Input: part model. Units: mm. Frame: model coordinates. Face numbers are marked on the shaded views. A direction names the side the tool comes from. Give positions to 0.01 mm unless a question says otherwise; leave off trailing zeros. Order: outer loops, then holes, each group sorted by start corner. A loop starts at its lowest first (then second) coordinate and runs counter-clockwise, first axis right, second up. Notation, with made-up numbers: M -17,-36.5 L -1,-36.5 A14 cw -1,-18.5 Z; hole C 40,53 d2. An arc over 180 degrees is marked long. Use a Markdown table: item, result.
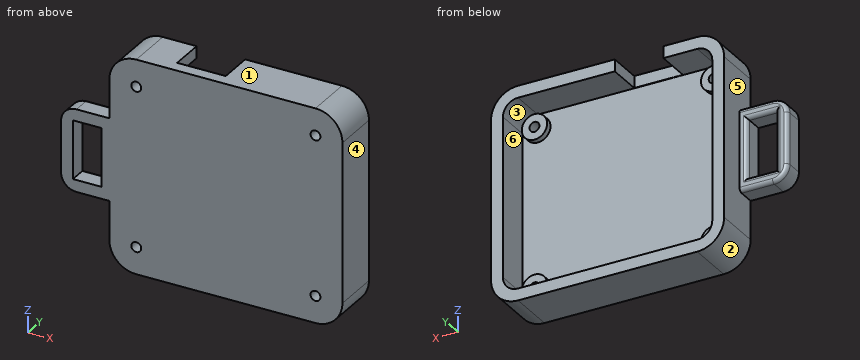
from build123d import *

# Parameters (mm, degrees)
BOSS_EXTRUDE1_DEPTH = 3
CUT_EXTRUDE1_REACH  = 77.661
SKETCH1_3_R         = 1.25
BOSS_EXTRUDE2_START = 8.86
BOSS_EXTRUDE2_DEPTH = 8.86
BOSS_EXTRUDE3_START = 1.5
SKETCH1_5_R         = 3.21
SKETCH1_5_R_2       = 1.25
BOSS_EXTRUDE3_DEPTH = 1.5
SKETCH2_W           = 12.28
SKETCH2_H           = 8.73
CUT_EXTRUDE2_DEPTH  = 3
SKETCH7_W           = 7.2
SKETCH7_H           = 14.75
BOSS_EXTRUDE6_DEPTH = 5
FILLET3_R           = 1


with BuildPart() as part:
    # Sketch1 → Boss-Extrude1 (new body)
    with BuildSketch(Plane(origin=(0, 0, 0), x_dir=(1, 0, 0), z_dir=(0, 1, 0))):
        with BuildLine():
            Line((3.81, 3), (49.09, 3))
            ThreePointArc((49.09, 3), (53.90539718, 1.00539718), (55.9, -3.81))
            Line((55.9, -3.81), (55.9, -44.09))
            ThreePointArc((55.9, -44.09), (53.90539718, -48.90539718), (49.09, -50.9))
            Line((49.09, -50.9), (3.81, -50.9))
            ThreePointArc((3.81, -50.9), (-1.00539718, -48.90539718), (-3, -44.09))
            Line((-3, -44.09), (-3, -3.81))
            ThreePointArc((-3, -3.81), (-1.00539718, 1.00539718), (3.81, 3))
        make_face()
    extrude(amount=-BOSS_EXTRUDE1_DEPTH)

    # Sketch1_3 → Cut-Extrude1 (cut, up to next)
    with BuildSketch(Plane(origin=(0, 0, 0), x_dir=(1, 0, 0), z_dir=(0, 1, 0)), mode=Mode.PRIVATE) as cut_extrude1_sk1:
        with Locations(Location((3.81, -3.81, 0), (0, 0, 270))):
            Circle(SKETCH1_3_R)
    cut_extrude1_tool1 = extrude(cut_extrude1_sk1.sketch, amount=-CUT_EXTRUDE1_REACH, mode=Mode.PRIVATE) & part.part
    # Sketch1_3 → Cut-Extrude1 (cut, up to next)
    with BuildSketch(Plane(origin=(0, 0, 0), x_dir=(1, 0, 0), z_dir=(0, 1, 0)), mode=Mode.PRIVATE) as cut_extrude1_sk2:
        with Locations(Location((3.81, -44.09, 0), (0, 0, 270))):
            Circle(SKETCH1_3_R)
    cut_extrude1_tool2 = extrude(cut_extrude1_sk2.sketch, amount=-CUT_EXTRUDE1_REACH, mode=Mode.PRIVATE) & part.part
    # Sketch1_3 → Cut-Extrude1 (cut, up to next)
    with BuildSketch(Plane(origin=(0, 0, 0), x_dir=(1, 0, 0), z_dir=(0, 1, 0)), mode=Mode.PRIVATE) as cut_extrude1_sk3:
        with Locations(Location((49.09, -44.09, 0), (0, 0, 270))):
            Circle(SKETCH1_3_R)
    cut_extrude1_tool3 = extrude(cut_extrude1_sk3.sketch, amount=-CUT_EXTRUDE1_REACH, mode=Mode.PRIVATE) & part.part
    # Sketch1_3 → Cut-Extrude1 (cut, up to next)
    with BuildSketch(Plane(origin=(0, 0, 0), x_dir=(1, 0, 0), z_dir=(0, 1, 0)), mode=Mode.PRIVATE) as cut_extrude1_sk4:
        with Locations(Location((49.09, -3.81, 0), (0, 0, 270))):
            Circle(SKETCH1_3_R)
    cut_extrude1_tool4 = extrude(cut_extrude1_sk4.sketch, amount=-CUT_EXTRUDE1_REACH, mode=Mode.PRIVATE) & part.part
    add(cut_extrude1_tool1.solids().sort_by_distance((3.81, 0, 3.81))[0], mode=Mode.SUBTRACT)
    add(cut_extrude1_tool2.solids().sort_by_distance((3.81, 0, 44.09))[0], mode=Mode.SUBTRACT)
    add(cut_extrude1_tool3.solids().sort_by_distance((49.09, 0, 44.09))[0], mode=Mode.SUBTRACT)
    add(cut_extrude1_tool4.solids().sort_by_distance((49.09, 0, 3.81))[0], mode=Mode.SUBTRACT)

    # Sketch1_4 → Boss-Extrude2 (add)
    with BuildSketch(Plane(origin=(0, 0, 0), x_dir=(1, 0, 0), z_dir=(0, 1, 0)).offset(BOSS_EXTRUDE2_START)):
        with BuildLine():
            ThreePointArc((-3, -3.81), (-1.00539718, 1.00539718), (3.81, 3))
            Line((3.81, 3), (49.09, 3))
            ThreePointArc((49.09, 3), (53.90539718, 1.00539718), (55.9, -3.81))
            Line((55.9, -3.81), (55.9, -44.09))
            ThreePointArc((55.9, -44.09), (53.90539718, -48.90539718), (49.09, -50.9))
            Line((49.09, -50.9), (3.81, -50.9))
            ThreePointArc((3.81, -50.9), (-1.00539718, -48.90539718), (-3, -44.09))
            Line((-3, -44.09), (-3, -3.81))
        make_face()
        with BuildLine():
            Line((52.9, -3.81), (52.9, -44.09))
            ThreePointArc((52.9, -44.09), (51.784076836, -46.784076836), (49.09, -47.9))
            Line((49.09, -47.9), (3.81, -47.9))
            ThreePointArc((3.81, -47.9), (1.115923164, -46.784076836), (0, -44.09))
            Line((0, -44.09), (0, -3.81))
            ThreePointArc((0, -3.81), (1.115923164, -1.115923164), (3.81, 0))
            Line((3.81, 0), (49.09, 0))
            ThreePointArc((49.09, 0), (51.784076836, -1.115923164), (52.9, -3.81))
        make_face(mode=Mode.SUBTRACT)
    extrude(amount=-BOSS_EXTRUDE2_DEPTH)

    # Sketch1_5 → Boss-Extrude3 (add)
    # profile 1 of 4: a face of its own
    with BuildSketch(Plane(origin=(0, 0, 0), x_dir=(1, 0, 0), z_dir=(0, 1, 0)).offset(BOSS_EXTRUDE3_START)):
        with Locations(Location((49.09, -3.81, 0), (0, 0, 90))):
            Circle(SKETCH1_5_R)
        with Locations(Location((49.09, -3.81, 0), (0, 0, 270))):
            Circle(SKETCH1_5_R_2, mode=Mode.SUBTRACT)
    # profile 2 of 4: a face of its own
    with BuildSketch(Plane(origin=(0, 0, 0), x_dir=(1, 0, 0), z_dir=(0, 1, 0)).offset(BOSS_EXTRUDE3_START)):
        with Locations(Location((49.09, -44.09, 0), (0, 0, 90))):
            Circle(SKETCH1_5_R)
        with Locations(Location((49.09, -44.09, 0), (0, 0, 270))):
            Circle(SKETCH1_5_R_2, mode=Mode.SUBTRACT)
    # profile 3 of 4: a face of its own
    with BuildSketch(Plane(origin=(0, 0, 0), x_dir=(1, 0, 0), z_dir=(0, 1, 0)).offset(BOSS_EXTRUDE3_START)):
        with Locations(Location((3.81, -44.09, 0), (0, 0, 90))):
            Circle(SKETCH1_5_R)
        with Locations(Location((3.81, -44.09, 0), (0, 0, 270))):
            Circle(SKETCH1_5_R_2, mode=Mode.SUBTRACT)
    # profile 4 of 4: a face of its own
    with BuildSketch(Plane(origin=(0, 0, 0), x_dir=(1, 0, 0), z_dir=(0, 1, 0)).offset(BOSS_EXTRUDE3_START)):
        with Locations(Location((3.81, -3.81, 0), (0, 0, 90))):
            Circle(SKETCH1_5_R)
        with Locations(Location((3.81, -3.81, 0), (0, 0, 270))):
            Circle(SKETCH1_5_R_2, mode=Mode.SUBTRACT)
    extrude(amount=-BOSS_EXTRUDE3_DEPTH)

    # Sketch2 → Cut-Extrude2 (cut)
    with BuildSketch(Plane.XY.offset(50.9)):
        with Locations((18.5, 4.5)):
            Rectangle(SKETCH2_W, SKETCH2_H)
    extrude(amount=-CUT_EXTRUDE2_DEPTH, mode=Mode.SUBTRACT)

    # Sketch7 → Boss-Extrude6 (add)
    with BuildSketch(Plane(origin=(0, -3, 0), x_dir=(-1, 0, 0), z_dir=(0, -1, 0))):
        with BuildLine():
            Line((3, -34.325), (11.3, -34.325))
            ThreePointArc((11.3, -34.325), (14.057716447, -33.182716447), (15.2, -30.425))
            Line((15.2, -30.425), (15.2, -17.475))
            ThreePointArc((15.2, -17.475), (14.057716447, -14.717283553), (11.3, -13.575))
            Line((11.3, -13.575), (3, -13.575))
            Line((3, -13.575), (3, -34.325))
        make_face()
        with Locations((8.6, -23.95)):
            Rectangle(SKETCH7_W, SKETCH7_H, mode=Mode.SUBTRACT)
    extrude(amount=-BOSS_EXTRUDE6_DEPTH)

    # Fillet3
    fillet3_edges = [part.edges().sort_by_distance(p)[0] for p in [
        (-7.15, 2, 13.575),
        (-14.057716447, 2, 14.717283553),
        (-15.2, 2, 23.95),
        (-14.057716447, 2, 33.182716447),
        (-7.15, 2, 34.325),
        (-12.2, 2, 23.95),
        (-8.6, 2, 16.575),
        (-5, 2, 23.95),
        (-8.6, 2, 31.325),
    ]]
    fillet(fillet3_edges, radius=FILLET3_R)


solid = part.part
1) First-contact query: pin 1 Ø2.5 at (y, z) = (6, 25.5) entering from -X; pin 2 Ø3 at (x, y) = (-7.5, 0) entering from +Z (3 decimals); pin 3 Ø2 at (x, z) = (39.5, 27.5) entering from +Y. Flat tips, straight axial feed; report the tip coordinate or a pass-through.
Response values:
| item | result |
|---|---|
| pin 1 | stops at x = -3 |
| pin 2 | stops at z = 34.325 |
| pin 3 | stops at y = 0 |
2) Mould query, pull axis X, two halves, no side actions, for the marked faces 1, 2 and 3. Classes: released by +X, released by -X, zero draft, split by the parting line, or undercut.
Response values:
| item | result |
|---|---|
| face 1 | zero draft |
| face 2 | released by -X |
| face 3 | undercut |
3) Cut plane A-A on z = 22. Return loops of the section in (x, y), and give its area (3 significant figures).
Response values:
| item | result |
|---|---|
| outline | M -15.2,-3 L -12.2,-3 L -12.2,1 A1 ccw -13.2,2 L -14.2,2 A1 ccw -15.2,1 Z; M -5,-3 L 55.9,-3 L 55.9,8.86 L 52.9,8.86 L 52.9,0 L 0,0 L 0,8.86 L -3,8.86 L -3,2 L -4,2 A1 ccw -5,1 Z |
| area | 254 mm² |
4) Cut plane B-B on x = 8. Return loops of the section in (y, z).
Response values:
| item | result |
|---|---|
| outline | M -3,-3 L 8.86,-3 L 8.86,0 L 0,0 L 0,47.9 L 8.86,47.9 L 8.86,50.9 L -3,50.9 Z |
5) Material intervals for line 1 (X direction, y = 0.1, z = 3.81); line 2 (X direction, y = -1.15, z = 3.81); line 3 (Z direction, x = 36, y = 0.5), sorted ascending. Write a range as from..to.
Response values:
| item | result |
|---|---|
| line 1 | x = -3..0, 0.6..2.56, 5.06..7.02, 45.88..47.84, 50.34..52.3, 52.9..55.9 |
| line 2 | x = -3..2.56, 5.06..47.84, 50.34..55.9 |
| line 3 | z = -3..0, 47.9..50.9 |
6) Reachability of the marked faces 4, 5 and 6 from +Z, -Z, +X, -X, +Y, -Y: full face, straight path, thin tool, end or side. Return the list, or none.
Response values:
| item | result |
|---|---|
| face 4 | +Z, -Z, +X, +Y, -Y |
| face 5 | -X, +Y |
| face 6 | +Y |
7) Cut plane C-C on y = 4.25. Return loops of the section in (x, z).
Response values:
| item | result |
|---|---|
| outline | M -3,3.81 A6.81 ccw 3.81,-3 L 49.09,-3 A6.81 ccw 55.9,3.81 L 55.9,44.09 A6.81 ccw 49.09,50.9 L 24.64,50.9 L 24.64,47.9 L 49.09,47.9 A3.81 cw 52.9,44.09 L 52.9,3.81 A3.81 cw 49.09,0 L 3.81,0 A3.81 cw 0,3.81 L 0,44.09 A3.81 cw 3.81,47.9 L 12.36,47.9 L 12.36,50.9 L 3.81,50.9 A6.81 ccw -3,44.09 Z |
